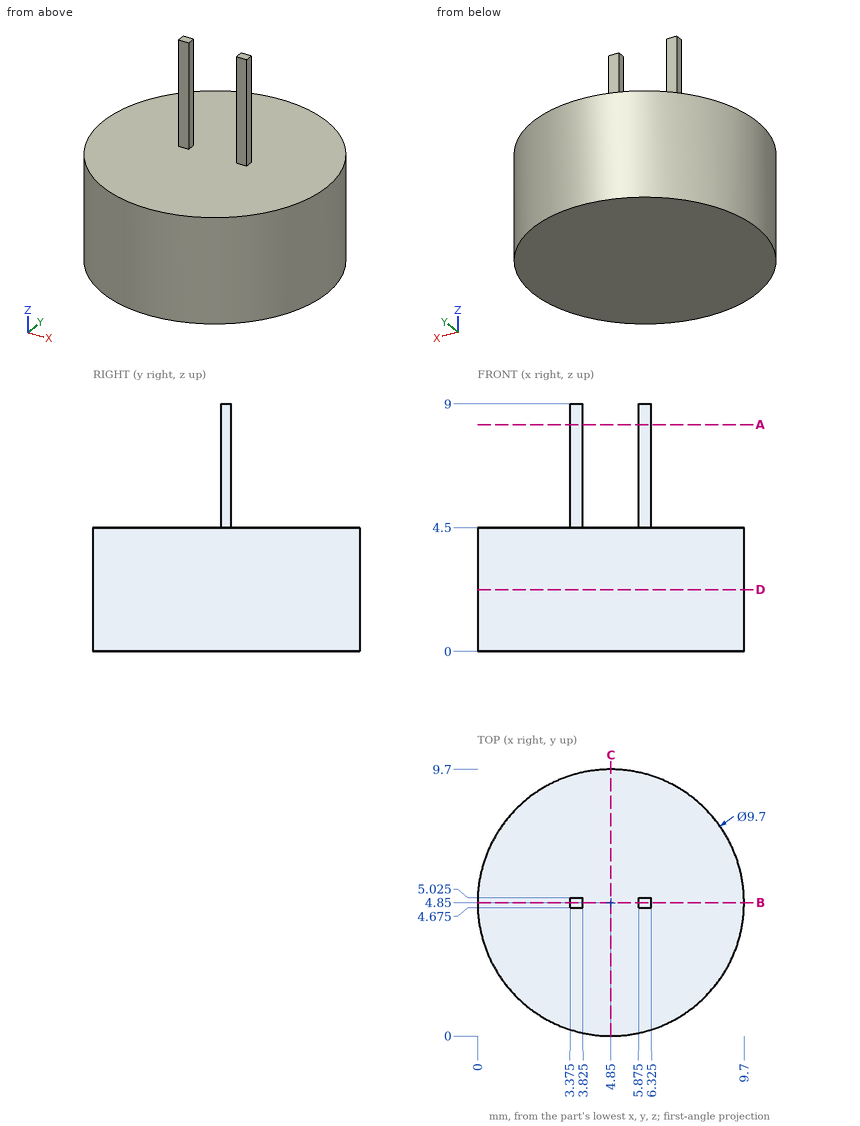
Verification items for this drawing (mm, ordinates from the low corner). Coordinates: 2 decimals unless noted, no trailing zeros. Write each loop counter-clockwise with the first axis right and the second up, starting at its lowest first coordinate (ties: lowest second). Pieces come first, ordered by that corner, then holes. Notation, with made-up numbers: M -7,-24 L 26,-24 A17 ccw 26,-5 Z; hole C 30.5,41 d1. An arc over 180 degrees is marked long. Use one line per item in the form item = value. Start each with the question number.
1) Go/stop test with flat-tipped pins: pin 1 Ø3 at (y, z) = (5.5, 7) entering from +X (3 decimals); pin 2 Ø1.5 at (y, z) = (6, 4) entering from +X; pin 3 Ø5 at (x, y) = (1.5, 2) entering from +Z. Record where each tip stops, or that it passes through.
2) Section check D-D on z = 2.25. Enter the section's corners in (x, y), and give its area (3 significant figures).
3) Section check B-B on y = 4.85. Enter the section's corners in (x, z) (3 decimals).
4) Section check C-C on x = 4.85. Enter the section's corners in (y, z).
5) Thickness scan on probe 1 along Z at (x, y) = (6.25, 7); probe 2 along Y at (x, z) = (4.75, 1); probe 3 along Y at (x, z) = (3.75, 1.5). Record the ranges inside material, lowest first. Write a range as from..to.
6) Section check A-A on z = 8.25. Enter the section's corners in (x, y) (3 decimals), and give its area (3 significant figures).
Responses:
q1.pin_1 = 6.325
q1.pin_2 = 9.68
q1.pin_3 = 4.5
q2.outline = C 4.85,4.85 d9.7
q2.area = 73.9 mm2
q3.outline = M 0,0 L 9.7,0 L 9.7,4.5 L 6.325,4.5 L 6.325,9 L 5.875,9 L 5.875,4.5 L 3.825,4.5 L 3.825,9 L 3.375,9 L 3.375,4.5 L 0,4.5 Z
q4.outline = M 0,0 L 9.7,0 L 9.7,4.5 L 0,4.5 Z
q5.probe_1 = 0..4.5
q5.probe_2 = 0..9.7
q5.probe_3 = 0.13..9.57
q6.outline = M 3.375,4.675 L 3.825,4.675 L 3.825,5.025 L 3.375,5.025 Z; M 5.875,4.675 L 6.325,4.675 L 6.325,5.025 L 5.875,5.025 Z
q6.area = 0.315 mm2
